```python
from build123d import *

# Parameters (mm, degrees)
SKETCH_1_R      = 2.5
EXTRUDE_1_DEPTH = 20
SKETCH_2_R      = 3.5
EXTRUDE_2_DEPTH = 2
FILLET_2_R      = 1


with BuildPart() as part:
    # 草图1 → 凸台-拉伸1 (new body)
    with BuildSketch(Plane.XY):
        Circle(SKETCH_1_R)
    extrude(amount=EXTRUDE_1_DEPTH)

    # 草图2 → 凸台-拉伸2 (add)
    with BuildSketch(Plane.XY.offset(20)):
        Circle(SKETCH_2_R)
    extrude(amount=EXTRUDE_2_DEPTH)

    # 圆角2
    fillet_2_edges = [part.edges().sort_by_distance(p)[0] for p in [
        (-3.5, 0, 20),
        (-3.5, 0, 22),
    ]]
    fillet(fillet_2_edges, radius=FILLET_2_R - 0.0001)  # a hair under: the kernel refuses the full size


solid = part.part
```
Design review of the part built by this model. Coordinates are the model's own, in mm. A direction names the side the tool comes from. Coordinates: 2 decimals unless noted, no trailing zeros. Loops run counter-clockwise (first coordinate to the right, second up) from the corner with the lowest first, then second, coordinate; pieces in that order, holes last. Notation, with made-up numbers: M 19.25,48.5 L 53.25,48.5 A6 cw 53.25,53.5 Z; hole C 28,-13 d9. An arc over 180 degrees is marked long. One line per question, with ' | ' between items.
(1) We need section C-C (z = 13.25). Give the boundary of the cut face in (x, y).
Filled in:
outline: C 0,0 d5
(2) Machinability: for faces 1 (the face through (-0.54, -2.44, 9.86)), 2 (the face through (0, 0, 0)), which of the approach directions +Z, -Z, +X, -X, +Y, -Y give a long, thin tool a straight path to every point of the face, cutting with its end or side? Answer none if there is none.
Filled in:
face 1: -Z | face 2: -Z, +X, -X, +Y, -Y
(3) Wall thickness on probe 1 along X at (y, z) = (-1.5, 12); probe 2 along Z at (x, y) = (-1, -3); probe 3 along Y at (x, z) = (-1.25, 13.5): over which ranges is each line inside the solid? List them lowest first.
Filled in:
probe 1: x = -2 to 2 | probe 2: z = 20.25 to 21.75 | probe 3: y = -2.17 to 2.17
(4) For pin 1 Ø3 at (x, z) = (-1, 8) entering from +Y; pin 2 Ø1.5 at (y, z) = (-2.5, 11.5) entering from +X, all flat-tipped, find the tip position at first contact; note any pin that passes through.
Filled in:
pin 1: stops at y = 2.5 | pin 2: stops at x = 1.79
